from build123d import *

# Parameters (mm, degrees)
SKETCH_R     = 1.6
PAD_DEPTH    = 20.5
SKETCH001_R  = 4.75
POCKET_DEPTH = 1


with BuildPart() as part:
    # Sketch → Pad (new body)
    with BuildSketch(Plane.XY):
        Polygon((0, 0), (0, 10.5), (6, 10.5), (6, 0), (6, -10.5), (0, -10.5), align=None)
        with Locations((3, 5.9)):
            Circle(SKETCH_R, mode=Mode.SUBTRACT)
        with Locations((3, -5.9)):
            Circle(SKETCH_R, mode=Mode.SUBTRACT)
    extrude(amount=PAD_DEPTH)

    # Sketch001 → Pocket (cut)
    with BuildSketch(Plane.YZ):
        with Locations((0, 10.25)):
            Circle(SKETCH001_R)
    extrude(amount=POCKET_DEPTH, mode=Mode.SUBTRACT)


solid = part.part
Geometry check sheet. Reference: the model listing, model coordinates, mm. Coordinates: 2 decimals unless noted, no trailing zeros. Order: outer loops, then holes, each group sorted by start corner. A loop starts at its lowest first (then second) coordinate and runs counter-clockwise, first axis right, second up. Notation, with made-up numbers: (54.25, 66.5) - (109.25, 66.5) arc R16 cw to (109.25, 75.5) - close; hole circle Ø8 at (24.5, 52). An arc over 180 degrees is marked (long way). One line per item, written item: value.
(1) Sectioned sample at A-A (x = 3). Enter the section's corners in (y, z), and give its area (3 significant figures).
Data:
outline: (-10.5, 0) - (-7.5, 0) - (-7.5, 20.5) - (-10.5, 20.5) - close; (-4.3, 0) - (4.3, 0) - (4.3, 20.5) - (-4.3, 20.5) - close; (7.5, 0) - (10.5, 0) - (10.5, 20.5) - (7.5, 20.5) - close
area: 299 mm^2
(2) Sectioned sample at B-B (y = 5.9). Enter the section's corners in (x, z).
Data:
outline: (0, 0) - (1.4, 0) - (1.4, 20.5) - (0, 20.5) - close; (4.6, 0) - (6, 0) - (6, 20.5) - (4.6, 20.5) - close
(3) Release check for a two-part mould opening along Z. For faces 1 (the face through (0.493, -1.03, 5.613)), 2 (the face through (1, 0, 10)), 3 (the face through (3, 0, 20.5)), 4 (the face through (0, 5, 10)) record: +Z half, -Z half, draft (parallel to the pull), parting line (faces both ways), or undercut.
Data:
face 1: undercut
face 2: undercut
face 3: +Z half
face 4: draft
(4) Sectioned sample at C-C (z = 10.25). Enter the section's corners in (x, y), and give its area (3 significant figures).
Data:
outline: (0, -10.5) - (6, -10.5) - (6, 10.5) - (0, 10.5) - (0, 4.75) - (1, 4.75) - (1, -4.75) - (0, -4.75) - close; hole circle Ø3.2 at (3, -5.9); hole circle Ø3.2 at (3, 5.9)
area: 100 mm^2
(5) Thickness scan on probe 1 along Y at (x, z) = (3, 4.5); probe 2 along Y at (x, z) = (4.1, 7.25); probe 3 along Z at (x, y) = (0.55, 0). Record the ranges inside material, lowest first. Write a range as from..to.
Data:
probe 1: y = -10.5..-7.5, -4.3..4.3, 7.5..10.5
probe 2: y = -10.5..-7.06, -4.74..4.74, 7.06..10.5
probe 3: z = 0..5.5, 15..20.5
(6) Sectioned sample at D-D (y = 0). Enter the section's corners in (x, z).
Data:
outline: (0, 0) - (6, 0) - (6, 20.5) - (0, 20.5) - (0, 15) - (1, 15) - (1, 5.5) - (0, 5.5) - close
